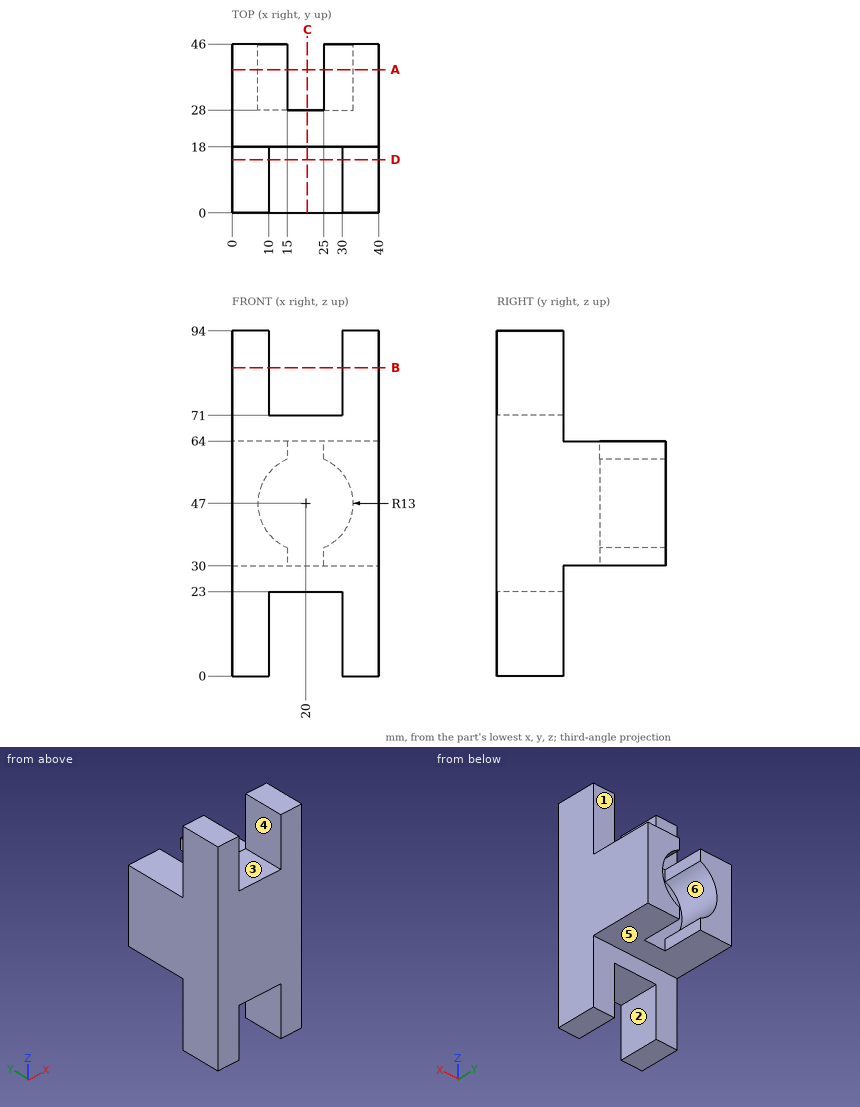
Could you check a few things on this drawing? It's one solid part, dimensions in mm from its lowest x, y, z. A direction names the side the tool comes from. Round coordinates to 2 decimals unless told otherwise and drop trailing zeros. Order: outer loops, then holes, each group sorted by start corner. A loop starts at its lowest first (then second) coordinate and runs counter-clockwise, first axis right, second up. Notation, with made-up numbers: (3, 65) -> (17, 65) arc R20 ccw to (17, 87) -> close; hole circle Ø5 at (45, 50.5). An arc over 180 degrees is marked (long way). One line per question, with ' | ' between items.
Q1. If I drill on line 1 (X direction, y = 40.5, z = 59); line 2 (Y direction, x = 8, z = 17.5); line 3 (Y direction, x = 17, z = 31.5), over which ranges is the centre line in solid material (lowest first)? Write a range as from..to.
Computed values:
line 1: 0..15, 25..40 | line 2: 0..18 | line 3: 0..28
Q2. If we section it at D-D on y = 14.5: Write out the boundary of the cut face in (x, z).
Computed values:
outline: (0, 0) -> (10, 0) -> (10, 23) -> (30, 23) -> (30, 0) -> (40, 0) -> (40, 94) -> (30, 94) -> (30, 71) -> (10, 71) -> (10, 94) -> (0, 94) -> close
Q3. Which directions (+Z, -Z, +X, -X, +Y, -Y) give clear straight access to the entire face, cutting with the end or side of a thin tool? Please do the marked faces 1, 2 and 3.
Computed values:
face 1: +Z, +X, -X, +Y | face 2: -Z, +Y, -Y | face 3: +Z, +Y, -Y
Q4. If we section it at C-C on x = 20.5: Write out the boundary of the cut face in (y, z), plus the area to 3 significant figures.
Computed values:
outline: (0, 23) -> (18, 23) -> (18, 30) -> (28, 30) -> (28, 64) -> (18, 64) -> (18, 71) -> (0, 71) -> close | area: 1,200 mm²
Q5. If we section it at B-B on z = 84: Write out the boundary of the cut face in (x, y), plus the area to 3 significant figures.
Computed values:
outline: (0, 0) -> (10, 0) -> (10, 18) -> (0, 18) -> close; (30, 0) -> (40, 0) -> (40, 18) -> (30, 18) -> close | area: 360 mm²
Q6. If we section it at A-A on y = 39: Write out the boundary of the cut face in (x, z), plus the area to 3 significant figures.
Computed values:
outline: (0, 30) -> (15, 30) -> (15, 35) arc R13 cw to (15, 59) -> (15, 64) -> (0, 64) -> close; (25, 30) -> (40, 30) -> (40, 64) -> (25, 64) -> (25, 59) arc R13 cw to (25, 35) -> close | area: 743 mm²
Q7. We'd pull the mould along Z, two halves only. Please class the marked faces 4, 5 and 6: released by +Z, released by -Z, zero draft, split by the parting line, or undercut.
Computed values:
face 4: zero draft | face 5: released by -Z | face 6: undercut
Q8. I'm going to push flat-ended pins straight in: pin 1 (9 mm diameter, centred on x = 14, z = 9, fed in from +Y); pin 2 (1 mm diameter, centred on x = 4, y = 36, fed in from -Z); pin 3 (5.5 mm diameter, centred on x = 17, y = 9.5, fed in from +Z). Where does each tip first touch, or does it pass through?
Computed values:
pin 1: y = 18 | pin 2: z = 30 | pin 3: z = 71
